The listing builds one solid part. Answer for the finished solid, in the listing's coordinates (mm). Face numbers are marked on the shaded views. Coordinates: 2 decimals unless noted, no trailing zeros. Order: outer loops, then holes, each group sorted by start corner. A loop starts at its lowest first (then second) coordinate and runs counter-clockwise, first axis right, second up. Notation, with made-up numbers: (-1.75, 32.5) -> (20.25, 32.5) arc R17 cw to (20.25, 47.5) -> close; hole circle Ø10 at (5, 32.25). An arc over 180 degrees is marked (long way). Write item = value, one per line.
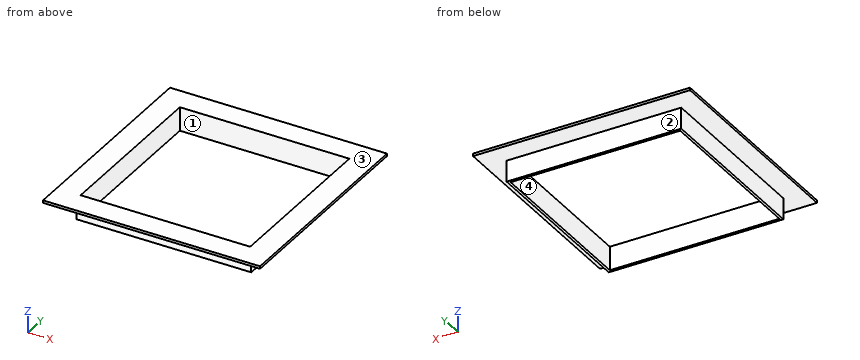
from build123d import *

# Parameters (mm, degrees)
SKETCH_W     = 400
SKETCH_H     = 60
PAD_DEPTH    = 200
SKETCH052_W  = 412
SKETCH052_H  = 50
PAD001_DEPTH = 206
SKETCH053_W  = 512
SKETCH053_H  = 512
PAD002_DEPTH = 6


with BuildPart() as body:
    # Sketch → Pad (new body, symmetric)
    with BuildSketch(Plane.XZ):
        with Locations((0, 30)):
            Rectangle(SKETCH_W, SKETCH_H)
    extrude(amount=PAD_DEPTH, both=True)


with BuildPart() as cut006:
    # Sketch052 → Pad001 (new body, symmetric)
    with BuildSketch(Plane.XZ):
        with Locations((0, 25)):
            Rectangle(SKETCH052_W, SKETCH052_H)
    extrude(amount=PAD001_DEPTH, both=True)

    # Sketch053 (on Face3 of Pad001) → Pad002 (join)
    with BuildSketch(Plane(origin=(0, 0, 50), x_dir=(-1, 0, 0), z_dir=(0, 0, 1))):
        Rectangle(SKETCH053_W, SKETCH053_H)
    extrude(amount=PAD002_DEPTH)

    # Cut006: cut Body
    add(body.part, mode=Mode.SUBTRACT)


solid = cut006.part
Q1. Find the intervals of material crossed by line 1 along X through (y, z) = (118, 38); line 2 along Y through (x, z) = (-167, 50.5), in increasing order.
The answers:
line_1 = -206 to -200, 200 to 206
line_2 = -256 to -200, 200 to 256
Q2. Each of these flat-tipped pins is pushed along its axis until it touches: pin 1 Ø25 at (y, z) = (95, 21.5) entering from +X; pin 2 Ø1 at (x, z) = (-182, 23.5) entering from +Y; pin 3 Ø25 at (x, z) = (-88.5, 36) entering from -Y. Where does it stop, or does it pass through?
The answers:
pin_1 = 206
pin_2 = 206
pin_3 = -206
Q3. The mould has two halves that part along Y. Classify the marked faces 1, 2, 3 and 4: released by +Y, released by -Y, zero draft, split by the parting line, or undercut.
The answers:
face_1 = undercut
face_2 = released by +Y
face_3 = zero draft
face_4 = undercut
Q4. Section B-B, the plane z = 6 is taken. Give the vertices of the cut face in (x, y).
The answers:
outline = (-206, -206) -> (206, -206) -> (206, 206) -> (-206, 206) -> close; hole (-200, -200) -> (200, -200) -> (200, 200) -> (-200, 200) -> close
Q5. Section A-A, the plane y = -121 is taken. Give the vertices of the cut face in (x, z), plus the area to 3 significant figures.
The answers:
outline = (-256, 50) -> (-206, 50) -> (-206, 0) -> (-200, 0) -> (-200, 56) -> (-256, 56) -> close; (200, 0) -> (206, 0) -> (206, 50) -> (256, 50) -> (256, 56) -> (200, 56) -> close
area = 1,270 mm2
